Part model, mm, in its own coordinate system. A direction names the side the tool comes from. Round coordinates to 2 decimals unless told otherwise and drop trailing zeros. Loops run counter-clockwise (first coordinate to the right, second up) from the corner with the lowest first, then second, coordinate; pieces in that order, holes last. Notation, with made-up numbers: M -4.75,44.25 L 18.25,44.25 A17 ccw 18.25,61.25 Z; hole C -6,34 d4. An arc over 180 degrees is marked long. Write each question's results on one line, items separated by ' | '.
from build123d import *

# Parameters (mm, degrees)
F1_DEPTH = 63.5
F0_W     = 24.4387735501
F0_H     = 19.05
F2_DEPTH = 25.4
F3_DEPTH = 12.7
F4_DEPTH = 25.4
F6_R     = 6.35


with BuildPart() as f1:
    # F0 (on Front) → F1 (new body, symmetric)
    with BuildSketch(Plane.XZ):
        Polygon((-41.275, 9.525), (-41.275, -9.525), (41.275, -9.525), (41.275, 9.525), (22.225, 9.525), align=None)
    extrude(amount=F1_DEPTH, both=True)

    # F0 (on Front) → F2 (join, symmetric)
    with BuildSketch(Plane.XZ):
        with BuildLine():
            Line((22.225, 9.525), (41.275, 9.525))
            Line((41.275, 9.525), (41.275, 27.0002))
            ThreePointArc((41.275, 27.0002), (45.9246798487, 38.2255201513), (57.15, 42.8752))
            Line((57.15, 42.8752), (60.325, 42.8752))
            Line((60.325, 42.8752), (60.325, 61.9252))
            Line((60.325, 61.9252), (57.15, 61.9252))
            ThreePointArc((57.15, 61.9252), (32.4542956671, 51.6959043329), (22.225, 27.0002))
            Line((22.225, 27.0002), (22.225, 9.525))
        make_face()
        with Locations((72.5443867751, 52.4002)):
            Rectangle(F0_W, F0_H)
    extrude(amount=F2_DEPTH, both=True)

    # F0 (on Front) → F3 (join, symmetric)
    with BuildSketch(Plane.XZ):
        with BuildLine():
            add(Edge.make_bspline(
                [(-41.275, 9.525), (-41.1736518145, 24.6508456767), (15.0934131816, 65.3959661722), (57.15, 61.9252)],
                knots=[0, 0, 0, 0, 111.5045361635, 111.5045361635, 111.5045361635, 111.5045361635], degree=3))
            Line((-41.275, 9.525), (22.225, 9.525))
            Line((22.225, 9.525), (22.225, 27.0002))
            ThreePointArc((22.225, 27.0002), (32.4542956671, 51.6959043329), (57.15, 61.9252))
        make_face()
    extrude(amount=F3_DEPTH, both=True)

    # F0 (on Front) → F4 (join, symmetric)
    with BuildSketch(Plane.XZ):
        with Locations((72.5443867751, 52.4002)):
            Rectangle(F0_W, F0_H)
    extrude(amount=F4_DEPTH, both=True)

    # F0 (on Front) → F5 (revolve)
    with BuildSketch(Plane.XZ):
        Polygon((84.7637735501, 66.675), (84.7637735501, 61.9252), (84.7637735501, 42.8752), (84.7637735501, 38.1), (111.125, 38.1), (111.125, 66.675), align=None)
    revolve(axis=Axis((84.7637735501, 0, 52.3875), (0, 0, 1)))

    # F6
    f6_edges = [f1.edges().sort_by_distance(p)[0] for p in [
        (-41.275, -63.5, 0),
        (41.275, -63.5, 0),
        (41.275, 63.5, 0),
        (-41.275, 63.5, 0),
    ]]
    fillet(f6_edges, radius=F6_R)


solid = f1.part
Item 1: Band-saw the part on C-C on y = -17.5. Give the cut face in (x, z) (3 decimals).
Filled sheet:
outline: M -41.275,-9.525 L 41.275,-9.525 L 41.275,27 A15.875 cw 57.15,42.875 L 65.049,42.875 L 65.049,38.1 L 104.478,38.1 L 104.478,66.675 L 65.049,66.675 L 65.049,61.925 L 57.15,61.925 A34.925 ccw 22.225,27 L 22.225,9.525 L -41.275,9.525 Z
Item 2: Which spindle directions (+Z, -Z, +X, -X, +Y, -Y) get a long thin tool onto all of the face, cutting with end or side? Do faces 1 (the flat face through (-2, -12.7, 32)), 2 (the flat face through (85, 0, 38.1)), 3 (the cylindrical face through (32.73, 18.96, 51.97)), 4 (the flat face through (58, 0, 42.875)), 5 (the flat face through (84, 0, 66.675)). Say none if no direction does.
Filled sheet:
face 1: +Z, -X, -Y | face 2: -Z, +X, +Y, -Y | face 3: +Z, -X, +Y | face 4: -Z | face 5: +Z, +X, -X, +Y, -Y
Item 3: Band-saw the part on B-B on x = 65.5. Give the cut face in (y, z) (3 decimals).
Filled sheet:
outline: M -25.4,42.875 L -17.995,42.875 L -17.995,38.1 L 17.995,38.1 L 17.995,42.875 L 25.4,42.875 L 25.4,61.925 L 17.995,61.925 L 17.995,66.675 L -17.995,66.675 L -17.995,61.925 L -25.4,61.925 Z
Item 4: Drop flat-ended pins along their axis: P1, Ø1.5, axis at y = 19, z = 13, coming from the -X side (3 decimals); P2, Ø10, axis at y = 16.5, z = 19, coming from the -X side; P3, Ø8, axis at x = 54, y = -12, coming from the -Z side. Give the stop position or say it passes through.
Filled sheet:
P1: x = 22.225 | P2: x = -39.06 | P3: z = 41.17
Item 5: Band-saw the part on A-A on z = 2. Give the cut face in (x, y) (3 decimals), and give its area (3 significant figures).
Filled sheet:
outline: M -41.275,-57.15 A6.35 ccw -34.925,-63.5 L 34.925,-63.5 A6.35 ccw 41.275,-57.15 L 41.275,57.15 A6.35 ccw 34.925,63.5 L -34.925,63.5 A6.35 ccw -41.275,57.15 Z | area: 10,400 mm^2
Item 6: Wall check: L1, parallel to X at y = 19.5, z = 21.5 (3 decimals); L2, parallel to Z at x = 0, y = 58 (3 decimals); L3, parallel to Y at x = 17, z = 11.5. Give the ranges that are in metal, low to high.
Filled sheet:
L1: 22.225 to 41.275 | L2: -9.525 to 9.525 | L3: -12.7 to 12.7
Item 7: Two-plate mould, pull along X, no slides. Class faces 6 (the cylindrical face through (39.464, -61.59, 0.133)), 7 (the flat face through (0, 63.5, 0)), 8 (the flat face through (58, 2, 61.925)): +X half, -X half, draft (parallel to the pull), parting line (faces both ways), or undercut.
Filled sheet:
face 6: +X half | face 7: draft | face 8: undercut
Item 8: Band-saw the part on D-D on x = 98.5. Give the cut face in (y, z) (3 decimals), and give its area (3 significant figures).
Filled sheet:
outline: M -22.5,38.1 L 22.5,38.1 L 22.5,66.675 L -22.5,66.675 Z | area: 1,290 mm^2
